Could you check a few things on this drawing? It's one solid part, dimensions in mm from its lowest x, y, z. A direction names the side the tool comes from. Coordinates: 2 decimals unless noted, no trailing zeros. Loops run counter-clockwise (first coordinate to the right, second up) from the corner with the lowest first, then second, coordinate; pieces in that order, holes last. Notation, with made-up numbers: M 6,83.5 L 27,83.5 A20 ccw 27,116.5 Z; hole C 5.5,82.25 d3. An arc over 180 degrees is marked long. Answer as a JSON object with one key per item and string values. Group by question number.
Item 1: If I drill on line 1 (Y direction, x = 35, z = 15.25); line 2 (Z direction, x = 15.5, y = 50.5); line 3 (Y direction, x = 5, z = 2.5), over which ranges is the centre line in solid material (lowest first)?
Item 2: I'm going to push flat-ended pins straight in: pin 1 Ø2 at (y, z) = (43, 17) entering from +X; pin 2 Ø7 at (x, y) = (35, 65) entering from +Z; pin 3 Ø3.5 at (x, y) = (65, 35) entering from -Z; pin 4 Ø8 at (y, z) = (41.5, 15) entering from -X. Where does each tip first touch, or does it pass through?
Item 3: Suppose I cut it at C-C (y = 65). Write out the boundary of the cut face in (x, z), then the cut area to 3 significant figures.
Item 4: Which directions (+Z, -Z, +X, -X, +Y, -Y) give clear straight access to the entire face, cutting with the end or side of a thin tool? Please do the marked faces 1 and 2.
Item 5: Suppose I cut it at A-A (y = 35). Write out the boundary of the cut face in (x, z).
Item 6: We'd pull the mould along Y, two halves only. Please class the marked faces 3, 4, 5 and 6: +Y half, -Y half, draft (parallel to the pull), parting line (faces both ways), or undercut.
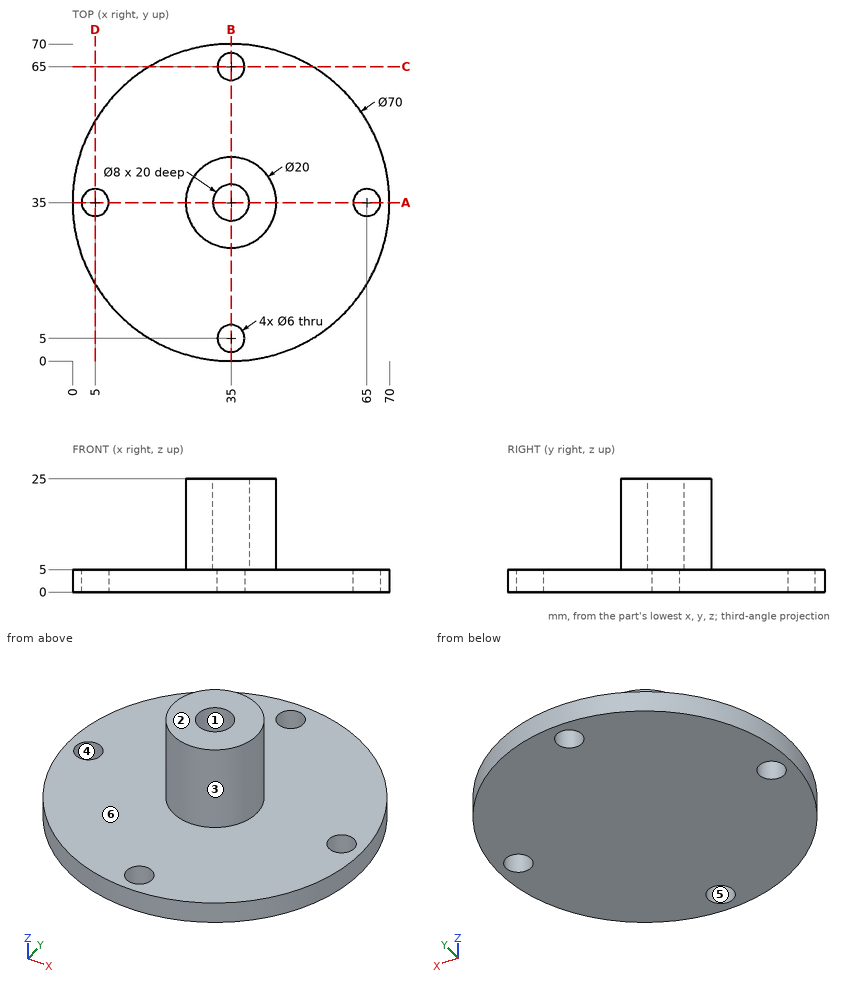
From the geometry:
{
 "1": {"line 1": "25 to 31, 39 to 45", "line 2": "0 to 5", "line 3": "16.97 to 32, 38 to 53.03"},
 "2": {"pin 1": "x = 42.14", "pin 2": "z = 5", "pin 3": "through", "pin 4": "x = 25.32"},
 "3": {"outline": "M 16.97,0 L 32,0 L 32,5 L 16.97,5 Z; M 38,0 L 53.03,0 L 53.03,5 L 38,5 Z", "area": "150 mm2"},
 "4": {"face 1": "+Z", "face 2": "+Z, +X, -X, +Y, -Y"},
 "5": {"outline": "M 0,0 L 2,0 L 2,5 L 0,5 Z; M 8,0 L 62,0 L 62,5 L 45,5 L 45,25 L 39,25 L 39,5 L 31,5 L 31,25 L 25,25 L 25,5 L 8,5 Z; M 68,0 L 70,0 L 70,5 L 68,5 Z"},
 "6": {"face 3": "parting line", "face 4": "undercut", "face 5": "undercut", "face 6": "draft"}
}
